Source: three-view drawing plus pictorial views. Frame: mm from the lowest corner of the part. A direction names the side the tool comes from. Coordinates: 2 decimals unless noted, no trailing zeros. Loops run counter-clockwise (first coordinate to the right, second up) from the corner with the lowest first, then second, coordinate; pieces in that order, holes last. Notation, with made-up numbers: M 55,7.25 L 65,7.25 A18 ccw 65,39.25 Z; hole C 11.5,-38.75 d4. An arc over 180 degrees is marked long. Use a Markdown table: item, result. Add a question column.
1. Section D-D on x = 47.5. Output: boundary loops of the cut face in (y, z).
2. Section B-B on x = 7.62. Output: boundary loops of the cut face in (y, z), then the cut area to 3 significant figures.
3. Line query: L1, parallel to Y at x = 22, z = 1.5; L2, parallel to Z at x = 42, y = 22.5; L3, parallel to Y at x = 11.5, z = 8.5. Output: solid intervals per line, ascending. Write a range as [from, to].
4. Draft query along Y for the marked faces 1, 2 and 3. Return one class per face: +Y half, -Y half, draft (parallel to the pull), parting line (faces both ways), or undercut.
5. Section A-A on y = 10.16. Output: boundary loops of the cut face in (x, z).
6. Pin query (flat end, axial travel): pin 1 (6 mm diameter, centred on x = 29, y = 10, fed in from -Z); pin 2 (8 mm diameter, centred on y = 10.16, z = 12.3, fed in from -X); pin 3 (1 mm diameter, centred on y = 25.5, z = 7, fed in from +X); pin 4 (4 mm diameter, centred on y = 20.16, z = 12.3, fed in from -X). Return the tip coordinate at first contact, or that it passes through.
7. Set-up query: the marked faces 4, 5, 6 and 7. Return all of +Z, -Z, +X, -X, +Y, -Y with unobstructed straight access to the full face (end or side cutting, diameter ignored); none if empty.
8. Section C-C on z = 7.62. Output: boundary loops of the cut face in (x, y).
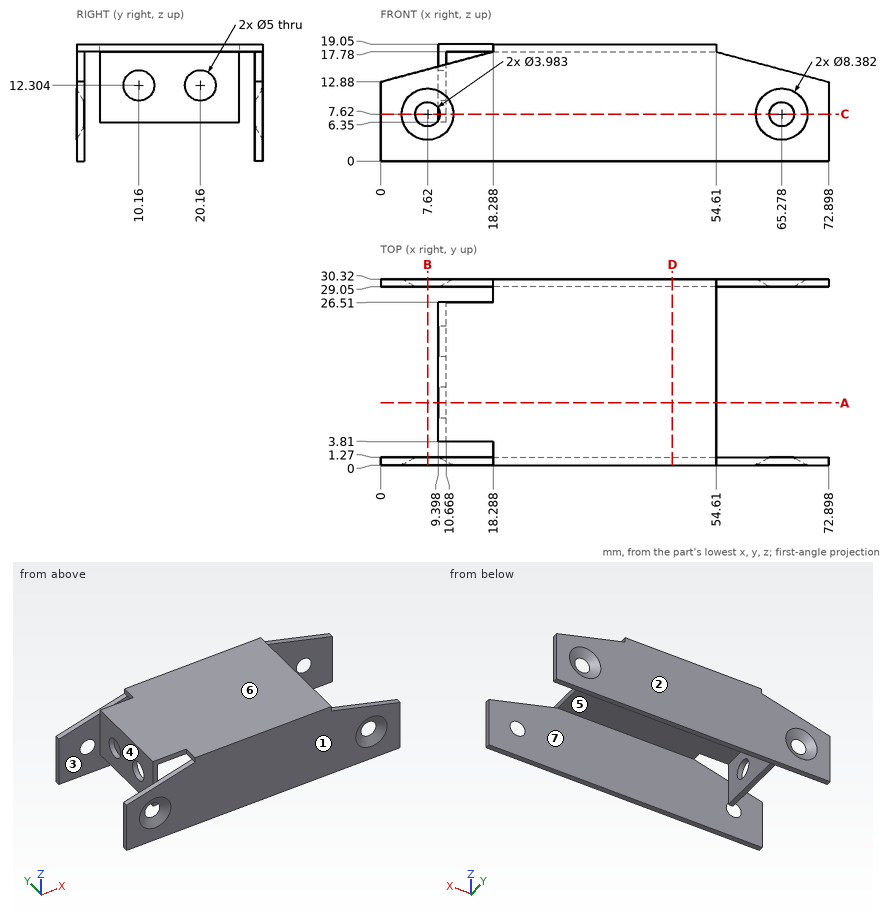
Answers below:
| question | item | result |
|---|---|---|
| 1 | outline | M 0,0 L 1.27,0 L 1.27,17.78 L 29.05,17.78 L 29.05,0 L 30.32,0 L 30.32,19.05 L 0,19.05 Z |
| 2 | outline | M 0,0 L 1.27,0 L 1.27,5.63 L 0,3.43 Z; M 0,11.81 L 1.27,9.61 L 1.27,14.92 L 0,14.92 Z; M 29.05,0 L 30.32,0 L 30.32,3.43 L 29.05,5.63 Z; M 29.05,9.61 L 30.32,11.81 L 30.32,14.92 L 29.05,14.92 Z |
| 2 | area | 22.2 mm² |
| 3 | L1 | y = [0, 1.27], [29.05, 30.32] |
| 3 | L2 | z = [17.78, 19.05] |
| 3 | L3 | y = [0.12, 1.27], [29.05, 30.2] |
| 4 | face 1 | -Y half |
| 4 | face 2 | +Y half |
| 4 | face 3 | undercut |
| 5 | outline | M 9.4,6.35 L 10.67,6.35 L 10.67,9.8 L 9.4,9.8 Z; M 9.4,14.8 L 10.67,14.8 L 10.67,17.78 L 54.61,17.78 L 54.61,19.05 L 9.4,19.05 Z |
| 6 | pin 1 | stops at z = 17.78 |
| 6 | pin 2 | stops at x = 9.4 |
| 6 | pin 3 | stops at x = 10.67 |
| 6 | pin 4 | passes through |
| 7 | face 4 | +Z, -Z, -X |
| 7 | face 5 | -Z, +X |
| 7 | face 6 | +Z, +X, -X, +Y, -Y |
| 7 | face 7 | -Z, +X, -X |
| 8 | outline | M 0,0 L 3.43,0 L 5.63,1.27 L 0,1.27 Z; M 0,29.05 L 5.63,29.05 L 3.43,30.32 L 0,30.32 Z; M 9.4,3.81 L 10.67,3.81 L 10.67,26.51 L 9.4,26.51 Z; M 9.61,1.27 L 11.81,0 L 61.09,0 L 63.29,1.27 Z; M 9.61,29.05 L 63.29,29.05 L 61.09,30.32 L 11.81,30.32 Z; M 67.27,1.27 L 69.47,0 L 72.9,0 L 72.9,1.27 Z; M 67.27,29.05 L 72.9,29.05 L 72.9,30.32 L 69.47,30.32 Z |
